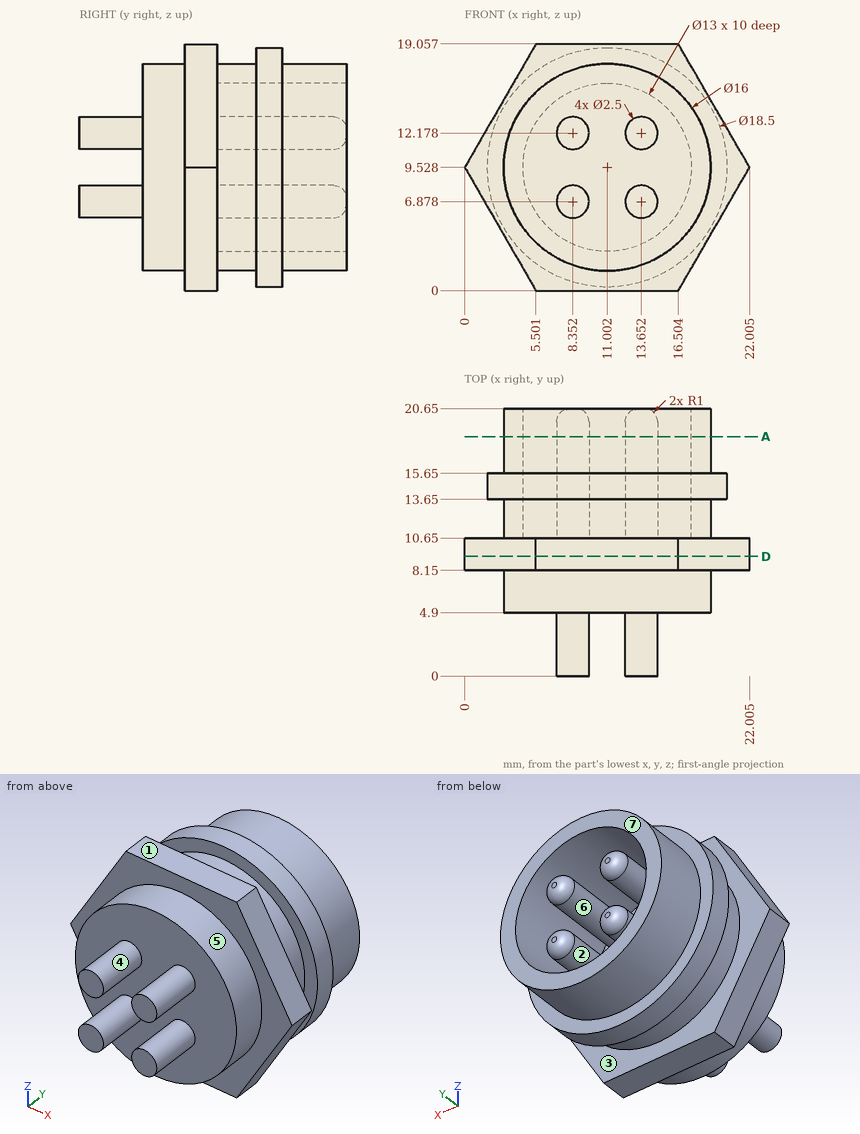
Can you work these out from the drawing? Everything is in mm from the part's minimum corner. A direction names the side the tool comes from. Coordinates: 2 decimals unless noted, no trailing zeros. Order: outer loops, then holes, each group sorted by start corner. A loop starts at its lowest first (then second) coordinate and runs counter-clockwise, first axis right, second up. Notation, with made-up numbers: (34, 78) -> (45, 78) arc R17 cw to (45, 106) -> close; hole circle Ø11 at (30, 25). An arc over 180 degrees is marked (long way). Use one line per item in the form item = value.
Q1. We'd pull the mould along X, two halves only. Please class the marked faces 5, 6 and 7: released by +X, released by -X, zero draft, split by the parting line, or undercut.
From the geometry:
face_5 = split by the parting line
face_6 = undercut
face_7 = zero draft
Q2. Will these pins go through, and if not, where does the flat tip stop? P1, Ø1, axis at y = 16, z = 8.5, coming from the -X side; P2, Ø6, axis at x = 18.5, z = 11, coming from the -Y side.
From the geometry:
P1 = 1.78
P2 = 4.9
Q3. Imagine slicing it at D-D, the plane y = 9.25. List the corners of the cut face in (x, z) for me (1 decimal).
From the geometry:
outline = (0, 9.5) -> (5.5, 0) -> (16.5, 0) -> (22, 9.5) -> (16.5, 19.1) -> (5.5, 19.1) -> close
Q4. I need wall thicknesses on L1, parallel to Z at x = 14.25, y = 15.75 (1 decimal); L2, parallel to Z at x = 8.25, y = 17.75 (1 decimal); L3, parallel to Y at x = 7, z = 4.75. Which ranges of each line are inside material? Lowest first, please.
From the geometry:
L1 = 2.2 to 3.9, 5.8 to 8, 11.1 to 13.3, 15.2 to 16.8
L2 = 2 to 3.6, 5.6 to 8.1, 10.9 to 13.4, 15.4 to 17
L3 = 4.9 to 10.65
Q5. Imagine slicing it at A-A, the plane y = 18.5. List the corners of the cut face in (x, z) for me.
From the geometry:
outline = circle Ø16 at (11, 9.53); circle Ø2.5 at (8.35, 6.88); circle Ø2.5 at (8.35, 12.18); circle Ø2.5 at (13.65, 6.88); circle Ø2.5 at (13.65, 12.18); hole circle Ø13 at (11, 9.53)
Q6. Which directions (+Z, -Z, +X, -X, +Y, -Y) give clear straight access to the entire face, cutting with the end or side of a thin tool? Please do the marked faces 1, 2, 3 and 4.
From the geometry:
face_1 = +Z, +X, -X, +Y, -Y
face_2 = +Y
face_3 = none
face_4 = -Y
